from build123d import *

# Parameters (mm, degrees)
BOSS_EXTRUDE1_DEPTH = 5.08
SKETCH2_R           = 1.143
CUT_EXTRUDE1_DEPTH  = 5.08
SKETCH3_R           = 1.016
CUT_EXTRUDE2_DEPTH  = 5.08


with BuildPart() as part:
    # Sketch1 → Boss-Extrude1 (new body)
    with BuildSketch(Plane.XY):
        Polygon((-75.921062447, -12.572076515), (-75.921062447, -10.410151662), (-50.521062447, -10.410151662), (-50.521062447, -19.300151662), (-53.061062447, -19.300151662), (-53.061062447, -12.572076515), align=None)
    extrude(amount=BOSS_EXTRUDE1_DEPTH)

    # Sketch2 → Cut-Extrude1 (cut)
    with BuildSketch(Plane(origin=(0, -10.410151662, 0), x_dir=(1, 0, 0), z_dir=(0, 1, 0))):
        with Locations((-73.381062447, -2.54)):
            Circle(SKETCH2_R)
    extrude(amount=-CUT_EXTRUDE1_DEPTH, mode=Mode.SUBTRACT)

    # Sketch3 → Cut-Extrude2 (cut)
    with BuildSketch(Plane(origin=(-50.521062447, 0, 0), x_dir=(0, 0, -1), z_dir=(1, 0, 0))):
        with Locations((-2.54, -14.728151662)):
            Circle(SKETCH3_R)
    extrude(amount=-CUT_EXTRUDE2_DEPTH, mode=Mode.SUBTRACT)


solid = part.part
Source: CAD feature listing. Evaluate the final solid. Frame: model axes, mm. A direction names the side the tool comes from. Round coordinates to 2 decimals unless told otherwise and drop trailing zeros. Order: outer loops, then holes, each group sorted by start corner. A loop starts at its lowest first (then second) coordinate and runs counter-clockwise, first axis right, second up. Notation, with made-up numbers: (72.25, 50.25) - (118.25, 50.25) arc R10 ccw to (118.25, 67.25) - close; hole circle Ø8 at (25, 50.25). An arc over 180 degrees is marked (long way). Use a Markdown table: item, result. Add a question column.
1. Set-up query: faces 4 (the flat face through (-53.061, -16, 3)), 5 (the flat face through (-75.921, -12, 3)). Return all of +Z, -Z, +X, -X, +Y, -Y with unobstructed straight access to the full face (end or side cutting, diameter ignored); none if empty.
2. Section query B-B (y = -15). Return the cut outline in (x, z).
3. Line query: probe 1 along X at (y, z) = (-11.45, 2.54); probe 2 along Y at (x, z) = (-52.2, 2.54); probe 3 along Y at (x, z) = (-66.25, 4.6). Output: solid intervals per line, ascending.
4. Mould query, pull axis Z, two halves, no side actions, for faces 1 (the cylindrical face through (-51.77, -15.72, 2.76)), 2 (the flat face through (-50.521, -16, 3)), 3 (the flat face through (-60, -12, 5.08)). Classes: +Z half, -Z half, draft (parallel to the pull), parting line (faces both ways), or undercut.
5. Section query C-C (x = -52.75). Return the cut outline in (y, z).
6. First-contact query: pin 1 (1.5 mm diameter, centred on y = -17.5, z = 2, fed in from -X); pin 2 (1.5 mm diameter, centred on x = -63, z = 3.5, fed in from -Y). Flat tips, straight axial feed; report the tip coordinate or a pass-through.
7. Section query A-A (z = 2.54). Return the cut outline in (x, y).
8. Section query D-D (y = -12.25). Return the cut outline in (x, z), then the cut area to 3 significant figures.
Derived:
| question | item | result |
|---|---|---|
| 1 | face 4 | +Z, -Z, -X, -Y |
| 1 | face 5 | +Z, -Z, -X, +Y, -Y |
| 2 | outline | (-53.06, 0) - (-50.52, 0) - (-50.52, 1.56) - (-53.06, 1.56) - close; (-53.06, 3.52) - (-50.52, 3.52) - (-50.52, 5.08) - (-53.06, 5.08) - close |
| 3 | probe 1 | -75.92 to -74.52, -72.24 to -50.52 |
| 3 | probe 2 | -19.3 to -15.74, -13.71 to -10.41 |
| 3 | probe 3 | -12.57 to -10.41 |
| 4 | face 1 | undercut |
| 4 | face 2 | draft |
| 4 | face 3 | +Z half |
| 5 | outline | (-19.3, 0) - (-10.41, 0) - (-10.41, 5.08) - (-19.3, 5.08) - close; hole circle Ø2.03 at (-14.73, 2.54) |
| 6 | pin 1 | x = -53.06 |
| 6 | pin 2 | y = -12.57 |
| 7 | outline | (-75.92, -12.57) - (-74.52, -12.57) - (-74.52, -10.41) - (-75.92, -10.41) - close; (-72.24, -12.57) - (-53.06, -12.57) - (-53.06, -13.71) - (-50.52, -13.71) - (-50.52, -10.41) - (-72.24, -10.41) - close; (-53.06, -19.3) - (-50.52, -19.3) - (-50.52, -15.74) - (-53.06, -15.74) - close |
| 8 | outline | (-75.92, 0) - (-50.52, 0) - (-50.52, 5.08) - (-75.92, 5.08) - close; hole circle Ø2.29 at (-73.38, 2.54) |
| 8 | area | 125 mm2 |
